Can you work these out from the model? Positions are in its coordinate system, mm. A direction names the side the tool comes from. Coordinates: 2 decimals unless noted, no trailing zeros. Write each loop counter-clockwise with the first axis right and the second up, starting at its lowest first coordinate (ties: lowest second). Pieces come first, ordered by that corner, then holes. Notation, with made-up numbers: (-1.75, 68) - (4.25, 68) arc R29 cw to (4.25, 89) - close; hole circle Ø8 at (52.5, 81.25). An arc over 180 degrees is marked (long way). Write each question's results on one line, items separated by ' | '. Start each with the question number.
```python
from build123d import *

# Parameters (mm, degrees)
F0_W      = 25.4
F0_H      = 24.1169882938
F1_DEPTH  = 2.54
F0_H_2    = 25.4
F2_W      = 2.9306858778
F2_H      = 25.4
F4_DEPTH  = 38.1
F3_W      = 2.9306774
F3_H      = 24.1169882938
F6_D      = 3.7084
F6_DEPTH  = 12.7
F6_TIP    = 1.1141157598
F8_D      = 3.7084
F8_DEPTH  = 12.7
F8_TIP    = 1.1141157598
F11_D     = 3.7084
F11_DEPTH = 12.7
F11_TIP   = 1.1141157598


with BuildPart() as f1:
    # F0 (on Front) → F1 (new body)
    with BuildSketch(Plane.XZ):
        with Locations((25.2723555684, -23.3813137747)):
            Rectangle(F0_W, F0_H)
    extrude(amount=F1_DEPTH)

    # F3 (on face) → F4, piece 2 (join)
    with BuildSketch(Plane.XZ.offset(2.54)):
        with Locations((36.5070168684, -23.3813137747)):
            Rectangle(F3_W, F3_H)
    extrude(amount=F4_DEPTH)

    # F8
    with Locations(Plane.XZ.offset(2.54)):
        with Locations((24.4828648865, -16.1586906761)):
            Hole(F8_D / 2, depth=F8_DEPTH)
            with Locations((0, 0, -(F8_DEPTH + F8_TIP / 2))):  # 118° drill point
                Cone(0, F8_D / 2, F8_TIP, mode=Mode.SUBTRACT)


with BuildPart() as f1b:
    # F0 (on Front) → F1, piece 2 (new body)
    with BuildSketch(Plane.XZ):
        with Locations((-56.0397792935, -31.5795045674)):
            Rectangle(F0_W, F0_H_2)
    extrude(amount=F1_DEPTH)

    # F2 (on face) → F4 (join)
    with BuildSketch(Plane.XZ.offset(2.54)):
        with Locations((-67.2744363546, -31.5795045674)):
            Rectangle(F2_W, F2_H)
    extrude(amount=F4_DEPTH)

    # F6
    with Locations(Plane.XZ.offset(2.54)):
        with Locations((-56.6043816507, -23.6014798284)):
            Hole(F6_D / 2, depth=F6_DEPTH)
            with Locations((0, 0, -(F6_DEPTH + F6_TIP / 2))):  # 118° drill point
                Cone(0, F6_D / 2, F6_TIP, mode=Mode.SUBTRACT)

    # F11
    with Locations(Plane.XZ.offset(2.54)):
        with Locations((-56.0724250972, -41.6174791753)):
            Hole(F11_D / 2, depth=F11_DEPTH)
            with Locations((0, 0, -(F11_DEPTH + F11_TIP / 2))):  # 118° drill point
                Cone(0, F11_D / 2, F11_TIP, mode=Mode.SUBTRACT)


solid = f1b.part
```
Q1. Thinking about a two-plate mould opening in Z: for faces 1 (the face through (-43.34, -1, -32)), 2 (the face through (-66, -14, -44.28)), 3 (the face through (-57.46, -1.252, -25.246)), 4 (the face through (-66, -14, -18.88)), which applies, pulls with the +Z half, pulls with the -Z half, needs draft (parallel to the pull), parting line crosses it, or undercut?
Q2. If we section it at A-A (z = -25): Please give me the cut outline in (x, y), then the cut area to 3 significant figures.
Q3. If we section it at D-D (y = -9.5): Please give me the cut outline in (x, z).
Q4. If we section it at B-B (x = -56.75): Please give me the cut outline in (y, z).
Q5. For faces 5 (the face through (-67, -40.64, -31)), 6 (the face through (-55, -2.54, -31)), which set-ups out of +Z, -Z, +X, -X, +Y, -Y let a thin tool reach every point of the face, with its end or its side?
Q6. If we section it at C-C (z = -31.5): Please give me the cut outline in (x, y).
Q7. I need wall thicknesses on line 1 along Y through (x, z) = (-51, -43); line 2 along X through (y, z) = (-6, -42.25). Which ranges of each line are inside material? Lowest first, please. Write a range as from..to.
Q8. I'm going to push flat-ended pins straight in: pin 1 Ø5 at (y, z) = (-8.5, -37.5) entering from +X; pin 2 Ø5 at (x, z) = (-48.5, -29.5) entering from -Y; pin 3 Ø2 at (x, z) = (-56.07, -41.62) entering from +Y. Where does each tip first touch, or does it pass through?
Answer list:
1) face 1: needs draft | face 2: pulls with the -Z half | face 3: undercut | face 4: pulls with the +Z half
2) outline: (-68.74, -40.64) - (-65.81, -40.64) - (-65.81, -2.54) - (-57.82, -2.54) - (-57.82, 0) - (-68.74, 0) - close; (-55.39, -2.54) - (-43.34, -2.54) - (-43.34, 0) - (-55.39, 0) - close | area: 170 mm2
3) outline: (-68.74, -44.28) - (-65.81, -44.28) - (-65.81, -18.88) - (-68.74, -18.88) - close
4) outline: (-2.54, -44.28) - (0, -44.28) - (0, -43.34) - (-2.54, -43.34) - close; (-2.54, -39.89) - (0, -39.89) - (0, -25.45) - (-2.54, -25.45) - close; (-2.54, -21.75) - (0, -21.75) - (0, -18.88) - (-2.54, -18.88) - close
5) face 5: +Z, -Z, +X, -X, -Y | face 6: +Z, -Z, +X, -Y
6) outline: (-68.74, -40.64) - (-65.81, -40.64) - (-65.81, -2.54) - (-43.34, -2.54) - (-43.34, 0) - (-68.74, 0) - close
7) line 1: y = -2.54..0 | line 2: x = -68.74..-65.81
8) pin 1: stops at x = -65.81 | pin 2: stops at y = -2.54 | pin 3: passes through
